Input: part model. Units: mm. Frame: model coordinates. Face numbers are marked on the shaded views. A direction names the side the tool comes from. Give positions to 0.01 mm unless a question says otherwise; leave off trailing zeros. Order: outer loops, then holes, each group sorted by start corner. A loop starts at its lowest first (then second) coordinate and runs counter-clockwise, first axis right, second up. Notation, with made-up numbers: M 13.5,4 L 60.5,4 A21 ccw 60.5,34 Z; hole C -27,4.25 d1. An arc over 180 degrees is marked long. Use a Markdown table: item, result.
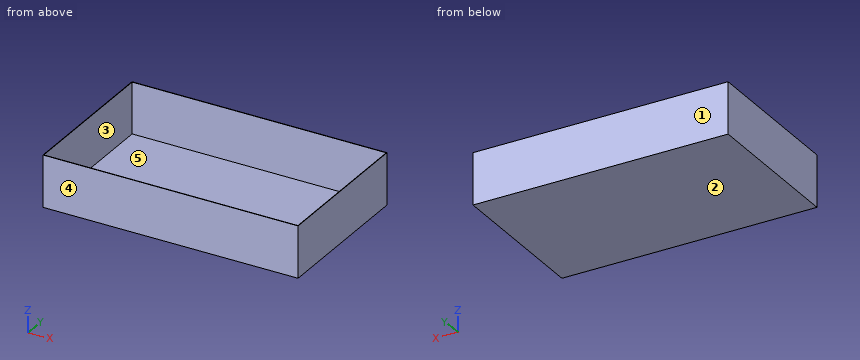
from build123d import *

# Parameters (mm, degrees)
F0_W     = 500
F0_H     = 300
F1_DEPTH = 1
F2_W     = 1
F2_H     = 1
F2_W_2   = 498
F2_H_2   = 298
F3_DEPTH = 100


with BuildPart() as f1:
    # F0 (on Top) → F1 (new body)
    with BuildSketch(Plane.XY):
        Rectangle(F0_W, F0_H)
    extrude(amount=F1_DEPTH)

    # F2 (on face) → F3 (join)
    with BuildSketch(Plane.XY.offset(1)):
        with Locations((-249.5, 149.5)):
            Rectangle(F2_W, F2_H)
        with Locations((0, 149.5)):
            Rectangle(F2_W_2, F2_H)
        with Locations((-249.5, 0)):
            Rectangle(F2_W, F2_H_2)
        with Locations((249.5, 149.5)):
            Rectangle(F2_W, F2_H)
        with Locations((-249.5, -149.5)):
            Rectangle(F2_W, F2_H)
        with Locations((0, -149.5)):
            Rectangle(F2_W_2, F2_H)
        with Locations((249.5, 0)):
            Rectangle(F2_W, F2_H_2)
        with Locations((249.5, -149.5)):
            Rectangle(F2_W, F2_H)
    extrude(amount=F3_DEPTH)


solid = f1.part
1) Cut plane A-A on x = 211. Return loops of the section in (y, z), and give its area (3 significant figures).
Response values:
| item | result |
|---|---|
| outline | M -150,0 L 150,0 L 150,101 L 149,101 L 149,1 L -149,1 L -149,101 L -150,101 Z |
| area | 500 mm² |
2) Mould query, pull axis Y, two halves, no side actions, for the marked faces 1, 2 and 3. Classes: released by +Y, released by -Y, zero draft, split by the parting line, or undercut.
Response values:
| item | result |
|---|---|
| face 1 | released by +Y |
| face 2 | zero draft |
| face 3 | undercut |
3) Material intervals for line 1 (X direction, y = -134.5, z = 8); line 2 (Y direction, x = 86, z = 41); line 3 (Z direction, x = 9, y = 118), sorted ascending. Write a range as from..to.
Response values:
| item | result |
|---|---|
| line 1 | x = -250..-249, 249..250 |
| line 2 | y = -150..-149, 149..150 |
| line 3 | z = 0..1 |
4) Cut plane C-C on z = 40.5. Return loops of the section in (x, y).
Response values:
| item | result |
|---|---|
| outline | M -250,-150 L 250,-150 L 250,150 L -250,150 Z; hole M -249,-149 L 249,-149 L 249,149 L -249,149 Z |
5) Cut plane B-B on y = 27.5. Return loops of the section in (x, z), and give its area (3 significant figures).
Response values:
| item | result |
|---|---|
| outline | M -250,0 L 250,0 L 250,101 L 249,101 L 249,1 L -249,1 L -249,101 L -250,101 Z |
| area | 700 mm² |
6) Reachability of the marked faces 4 and 5 from +Z, -Z, +X, -X, +Y, -Y: full face, straight path, thin tool, end or side. Return the list, or none.
Response values:
| item | result |
|---|---|
| face 4 | +Z, -Z, +X, -X, -Y |
| face 5 | +Z |
7) First-contact query: pin 1 Ø8 at (x, y) = (158, 74) entering from +Z. Flat tip, straight axial feed; report the tip coordinate or a pass-through.
Response values:
| item | result |
|---|---|
| pin 1 | stops at z = 1 |
